Geometry check sheet. Reference: the model listing, model coordinates, mm. A direction names the side the tool comes from. Round coordinates to 2 decimals unless told otherwise and drop trailing zeros. Write each loop counter-clockwise with the first axis right and the second up, starting at its lowest first coordinate (ties: lowest second). Pieces come first, ordered by that corner, then holes. Notation, with made-up numbers: (-10, 45.25) -> (47, 45.25) arc R16 cw to (47, 55.25) -> close; hole circle Ø2 at (9, 10.25). An arc over 180 degrees is marked (long way). Use a Markdown table: item, result.
```python
from build123d import *

# Parameters (mm, degrees)
F1_DEPTH = 500
F3_DEPTH = 100


with BuildPart() as f1:
    # F0 (on Front) → F1 (new body)
    with BuildSketch(Plane.XZ):
        Polygon((0, 16.431924), (-8.5, 16.431924), (-8.5, 13.145539), (-2.30047, 13.145539), (-2.30047, -17.568076), (0, -17.568076), (2.30047, -17.568076), (2.30047, 13.145539), (8.5, 13.145539), (8.5, 16.431924), align=None)
    extrude(amount=F1_DEPTH)

    # F2 (on face) → F3 (cut)
    with BuildSketch(Plane.YZ.offset(2.30047)):
        Polygon((0, -17.568076), (-500, 13.145539), (-500, -17.568076), align=None)
    extrude(amount=-F3_DEPTH, mode=Mode.SUBTRACT)


solid = f1.part
```
(1) Access from +Z, -Z, +X, -X, +Y, -Y to the whole of each face (thin tool, end or side, straight path). Record for faces 1 (the face through (2.3, -135, 4)), 2 (the face through (-2.3, -191, 1)), 3 (the face through (0, -246, 16.432)).
A:
| item | result |
|---|---|
| face 1 | -Z, +X, +Y, -Y |
| face 2 | -Z, -X, +Y, -Y |
| face 3 | +Z, +X, -X, +Y, -Y |
(2) Section check A-A on y = -156. Record the cut outline in (x, z).
A:
| item | result |
|---|---|
| outline | (-8.5, 13.15) -> (-2.3, 13.15) -> (-2.3, -7.99) -> (2.3, -7.99) -> (2.3, 13.15) -> (8.5, 13.15) -> (8.5, 16.43) -> (-8.5, 16.43) -> close |
(3) Section check D-D on y = -423. Record the cut outline in (x, z).
A:
| item | result |
|---|---|
| outline | (-8.5, 13.15) -> (-2.3, 13.15) -> (-2.3, 8.42) -> (2.3, 8.42) -> (2.3, 13.15) -> (8.5, 13.15) -> (8.5, 16.43) -> (-8.5, 16.43) -> close |
(4) Thickness scan on line 1 (Z direction, x = 4, y = -421.5); line 2 (X direction, y = -30, z = 11.5); line 3 (Z direction, x = 1.5, y = -293). Record the ranges inside material, lowest first.
A:
| item | result |
|---|---|
| line 1 | z = 13.15 to 16.43 |
| line 2 | x = -2.3 to 2.3 |
| line 3 | z = 0.43 to 16.43 |
(5) Section check C-C on z = -13. Record the cut outline in (x, y), plus the area to 3 significant figures.
A:
| item | result |
|---|---|
| outline | (-2.3, -74.37) -> (2.3, -74.37) -> (2.3, 0) -> (-2.3, 0) -> close |
| area | 342 mm2 |
(6) Gauge pin test, flat ends, axial feed: pin 1 Ø3 at (x, y) = (-6.5, -305.5) entering from -Z; pin 2 Ø1.5 at (x, y) = (2, -389) entering from -Z; pin 3 Ø6 at (x, y) = (-4, -436) entering from -Z; pin 4 Ø1 at (x, z) = (-1, 7) entering from +Y. Record the tip position at first contact, or that the pin passes through.
A:
| item | result |
|---|---|
| pin 1 | stops at z = 13.15 |
| pin 2 | stops at z = 6.28 |
| pin 3 | stops at z = 9.06 |
| pin 4 | stops at y = 0 |
(7) Section check B-B on x = -5.5. Record the cut outline in (y, z).
A:
| item | result |
|---|---|
| outline | (-500, 13.15) -> (0, 13.15) -> (0, 16.43) -> (-500, 16.43) -> close |
